Design review of the part shown in the three views and the two pictorial views. Dimensions are in mm from the part's minimum x, y and z. A direction names the side the tool comes from. Coordinates: 2 decimals unless noted, no trailing zeros. Order: outer loops, then holes, each group sorted by start corner. A loop starts at its lowest first (then second) coordinate and runs counter-clockwise, first axis right, second up. Notation, with made-up numbers: (79.25, 86.5) -> (137.25, 86.5) arc R21 ccw to (137.25, 95.5) -> close; hole circle Ø10 at (88.25, -34.5). An arc over 180 degrees is marked (long way). Write item = value, one per line. Start each with the question number.
1) Consider section A-A on x = 12.7. Give the boundary of the cut face in (y, z) (1 decimal), and give its area (3 significant figures).
2) Wall thickness on probe 1 along Z at (x, y) = (12.7, 5.25); probe 2 along Y at (x, z) = (1.25, 31.5) (3 decimals); probe 3 along Z at (x, y) = (2, 35): over which ranges is each line inside the solid? List them lowest first. Write a range as [from, to].
3) Consider section B-B on z = 22.86. Give the boundary of the cut face in (x, y) (1 decimal), and give its area (3 significant figures).
4) Consider section D-D on x = 23. Give the boundary of the cut face in (y, z) (3 decimals).
5) Insertion check: pin 1 Ø8.5 at (x, z) = (12.7, 22.86) entering from -Y; pin 2 Ø1 at (x, y) = (21, 21) entering from +Z; pin 3 Ø12.5 at (x, z) = (13, 29.5) entering from +Y (3 decimals). Each pin has a flat end and moves straight along its axis. Give the tip position at first contact, or say it passes through.
6) Draft analysis for pull direction Z (two halves, no side actions). For the marked faces 1, 2, 3 and 4, state which applies: +Z half, -Z half, draft (parallel to the pull), parting line (faces both ways), or undercut.
7) Consider section C-C on y = 12.5. Give the boundary of the cut face in (x, z) (1 decimal), and give its area (3 significant figures).
8) Machinability: for the marked faces 5 and 6, which of the approach directions +Z, -Z, +X, -X, +Y, -Y give a long, thin tool a straight path to every point of the face, cutting with its end or side? Answer none if there is none.
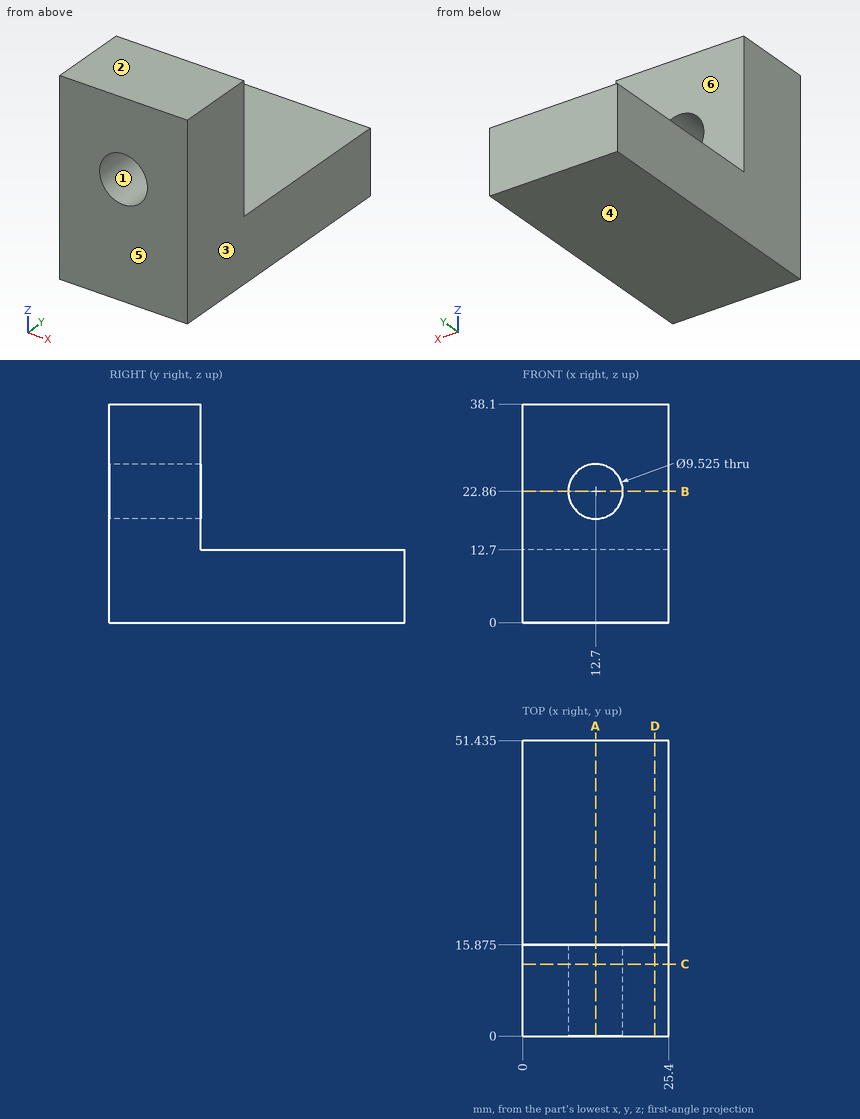
Answer sheet:
q1.outline = (0, 0) -> (51.4, 0) -> (51.4, 12.7) -> (15.9, 12.7) -> (15.9, 18.1) -> (0, 18.1) -> close; (0, 27.6) -> (15.9, 27.6) -> (15.9, 38.1) -> (0, 38.1) -> close
q1.area = 905 mm2
q2.probe_1 = [0, 18.1], [27.62, 38.1]
q2.probe_2 = [0, 15.875]
q2.probe_3 = [0, 12.7]
q3.outline = (0, 0) -> (7.9, 0) -> (7.9, 15.9) -> (0, 15.9) -> close; (17.5, 0) -> (25.4, 0) -> (25.4, 15.9) -> (17.5, 15.9) -> close
q3.area = 252 mm2
q4.outline = (0, 0) -> (51.435, 0) -> (51.435, 12.7) -> (15.875, 12.7) -> (15.875, 38.1) -> (0, 38.1) -> close
q5.pin_1 = through
q5.pin_2 = 12.7
q5.pin_3 = 15.875
q6.face_1 = undercut
q6.face_2 = +Z half
q6.face_3 = draft
q6.face_4 = -Z half
q7.outline = (0, 0) -> (25.4, 0) -> (25.4, 38.1) -> (0, 38.1) -> close; hole circle Ø9.5 at (12.7, 22.9)
q7.area = 896 mm2
q8.face_5 = +Z, -Z, +X, -X, -Y
q8.face_6 = +Z, +X, -X, +Y
